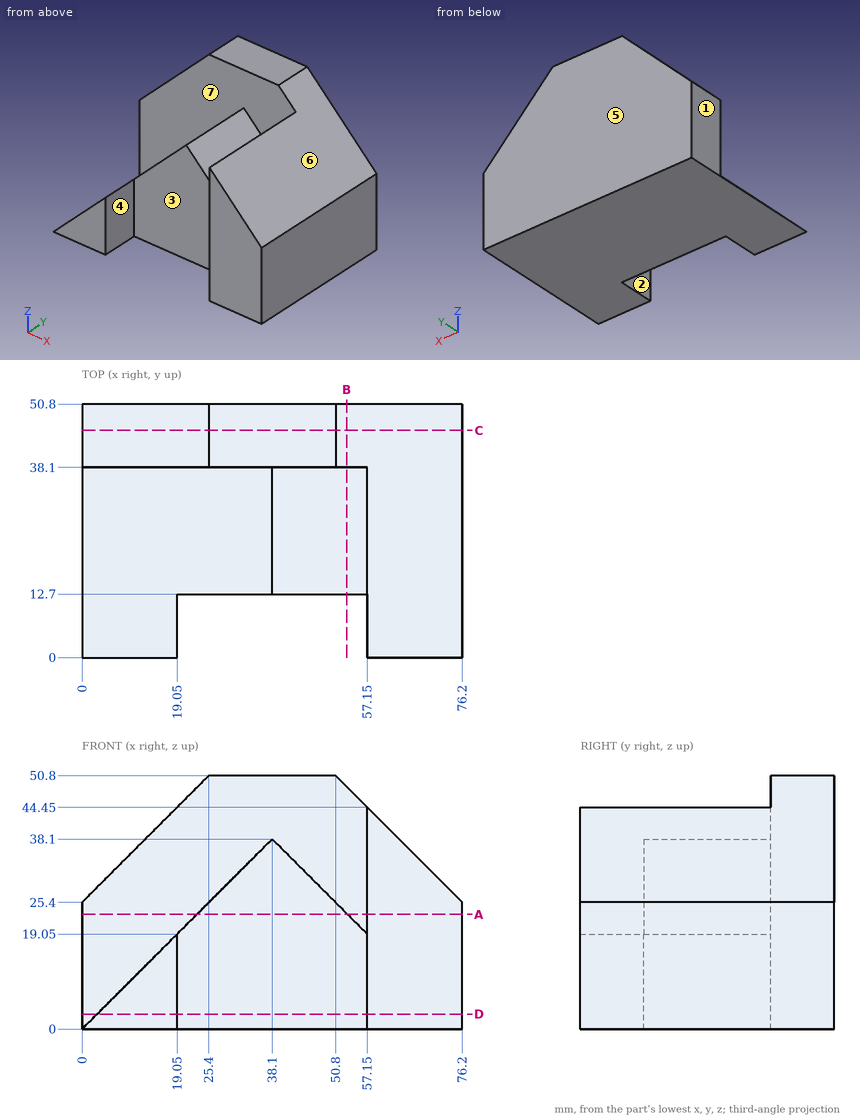
For this review, use the dimensioned drawing (mm, ordinates from the lowest corner) and the shaded views. A direction names the side the tool comes from. Round coordinates to 2 decimals unless told otherwise and drop trailing zeros. Write each loop counter-clockwise with the first axis right and the second up, starting at its lowest first coordinate (ties: lowest second). Pieces come first, ordered by that corner, then holes. Notation, with made-up numbers: M 29,75 L 52,75 A17 ccw 52,89 Z; hole C 5,-19 d6. An arc over 180 degrees is marked long. Answer as CSV lines item,"result". Start each with the question number.
Q1. Consider section A-A, the plane z = 23. Give the boundary of the cut face in (x, y).
Q2. Clearance check with flat-ended pins moving along their axes: P1, Ø8, axis at y = 28.5, z = 41.5, coming from the -X side; P2, Ø6, axis at x = 56.5, y = 25.5, coming from the +Z side; P3, Ø1, axis at y = 18.5, z = 40.5, coming from the +X side. State where each tip first meets the part, or that it passes through.
Q3. Consider section C-C, the plane y = 45.5. Give the boundary of the cut face in (x, z).
Q4. Consider section D-D, the plane z = 3. Give the boundary of the cut face in (x, y), then the cut area to 3 significant figures.
Q5. Consider section B-B, the plane x = 53. Give the boundary of the cut face in (y, z), then the cut area to 3 significant figures.
Q6. Wall thickness on line 1 along Y through (x, z) = (8, 20.5); line 2 along X through (y, z) = (15, 22.5); line 3 along X through (y, z) = (14.5, 24): over which ranges is each line inside the solid? List them lowest first.
Q7. Tool access review of the marked faces 1, 2 and 3: name each direction out of +Z, -Z, +X, -X, +Y, -Y from which nothing blocks a thin tool from reaching the whole face with its end or side.
Q8. The part is to be moulded in two halves that separate along X. For the marked faces 4, 5, 6 and 7, say which applies: +X half, -X half, draft (parallel to the pull), parting line (faces both ways), or undercut.
Result set:
1,outline,"M 0,38.1 L 23,38.1 L 23,12.7 L 53.2,12.7 L 53.2,38.1 L 57.15,38.1 L 57.15,0 L 76.2,0 L 76.2,50.8 L 0,50.8 Z"
2,P1,"stops at x = 37.5"
2,P2,"stops at z = 44.45"
2,P3,"stops at x = 61.6"
3,outline,"M 0,0 L 76.2,0 L 76.2,25.4 L 50.8,50.8 L 25.4,50.8 L 0,25.4 Z"
4,outline,"M 0,38.1 L 3,38.1 L 3,0 L 19.05,0 L 19.05,12.7 L 57.15,12.7 L 57.15,0 L 76.2,0 L 76.2,50.8 L 0,50.8 Z"
4,area,"3,270 mm²"
5,outline,"M 12.7,0 L 50.8,0 L 50.8,48.6 L 38.1,48.6 L 38.1,23.2 L 12.7,23.2 Z"
5,area,"1,210 mm²"
6,line 1,"y = 38.1 to 50.8"
6,line 2,"x = 22.5 to 53.7, 57.15 to 76.2"
6,line 3,"x = 24 to 52.2, 57.15 to 76.2"
7,face 1,"+Z, -Z, -X, +Y, -Y"
7,face 2,"+Z, -Y"
7,face 3,"+Z, -Z, -Y"
8,face 4,"undercut"
8,face 5,"draft"
8,face 6,"+X half"
8,face 7,"undercut"
